from build123d import *

# Parameters (mm, degrees)
F2_W      = 200
F2_H      = 529.5
F2_H_2    = 170
F2_H_3    = 529.5044031185
F3_DEPTH  = 60
F4_R      = 260
F5_DEPTH  = 90
F6_R      = 170
F7_DEPTH  = 25
F8_R      = 280
F9_DEPTH  = 15
F10_R     = 111
F11_DEPTH = 100
F12_R     = 150
F13_DEPTH = 8
F14_R     = 5
F15_DEPTH = 25
F16_R     = 100
F17_DEPTH = 200
F18_R     = 50
F19_DEPTH = 1000
F20_R     = 112.5
F20_R_2   = 99
F21_DEPTH = 100
F22_R     = 45
F23_DEPTH = 850
F25_R     = 100
F26_DEPTH = 10
F27_R     = 64.1521691024
F27_R_2   = 45
F28_DEPTH = 15
F29_R     = 9
F30_DEPTH = 25
F31_R     = 32.5
F32_DEPTH = 850
F34_R     = 82.5
F34_R_2   = 7
F35_DEPTH = 10
F36_R     = 50
F37_DEPTH = 25


with BuildPart() as f1:
    # F0 (on Front) → F1 (revolve)
    with BuildSketch(Plane.XZ):
        Polygon((0, 1515), (0, 0), (750, 0), (768.5, 0), (768.5, 5), (750, 5), (750, 1505), (773, 1505), (773, 1515), (750, 1515), align=None)
    revolve(axis=Axis((0, 0, 757.5), (0, 0, 1)))

    # F2 (on face) → F3 (join)
    with BuildSketch(Plane.XY.offset(1515)):
        Polygon((-100, 766.5), (-140, 766.5), (-140, -766.5), (-100, -766.5), (-100, -694.5), (100, -694.5), (100, -766.4955968815), (140, -766.4955968815), (140, 766.5044031185), (100, 766.5044031185), (100, 694.5044031185), (-100, 694.5044031185), align=None)
        with Locations((0, -389.75)):
            Rectangle(F2_W, F2_H, mode=Mode.SUBTRACT)
        Rectangle(F2_W, F2_H_2, mode=Mode.SUBTRACT)
        with Locations((0, 389.7522015592)):
            Rectangle(F2_W, F2_H_3, mode=Mode.SUBTRACT)
    extrude(amount=F3_DEPTH)

    # F4 (on face) → F5 (join)
    with BuildSketch(Plane.XY.offset(1515)):
        with Locations((-445, -50)):
            Circle(F4_R)
    extrude(amount=F5_DEPTH)

    # F6 (on face) → F7 (join)
    with BuildSketch(Plane.XY.offset(1515)):
        with Locations((-350, 425)):
            Circle(F6_R)
    extrude(amount=F7_DEPTH)

    # F8 (on face) → F9 (join)
    with BuildSketch(Plane.XY.offset(1605)):
        with Locations((-445, -50)):
            Circle(F8_R)
    extrude(amount=F9_DEPTH)

    # F10 (on face) → F11 (join)
    with BuildSketch(Plane.XY.offset(1515)):
        with Locations((350, 425)):
            Circle(F10_R)
    extrude(amount=F11_DEPTH)

    # F12 (on face) → F13 (join)
    with BuildSketch(Plane.XY.offset(1615)):
        with Locations((350, 425)):
            Circle(F12_R)
    extrude(amount=F13_DEPTH)

    # F14 (on face) → F15 (cut)
    with BuildSketch(Plane.XY.offset(1623)):
        with Locations((349.8037939217, 554.9998519352)):
            Circle(F14_R)
        with Locations((220.0001480648, 424.8037939217)):
            Circle(F14_R)
        with Locations((350.1962060783, 295.0001480648)):
            Circle(F14_R)
        with Locations((479.9998519352, 425.1962060783)):
            Circle(F14_R)
    extrude(amount=-F15_DEPTH, mode=Mode.SUBTRACT)

    # F16 (on face) → F17 (cut)
    with BuildSketch(Plane.XY.offset(1623)):
        with Locations((350, 425)):
            Circle(F16_R)
    extrude(amount=-F17_DEPTH, mode=Mode.SUBTRACT)

    # F18 (on face) → F19 (cut)
    with BuildSketch(Plane.XY.offset(1515)):
        Circle(F18_R)
    extrude(amount=-F19_DEPTH, mode=Mode.SUBTRACT)

    # F20 (on face) → F21 (join)
    with BuildSketch(Plane.XY.offset(1515)):
        with Locations((-315, -451)):
            Circle(F20_R)
        with Locations((-315, -451)):
            Circle(F20_R_2, mode=Mode.SUBTRACT)
    extrude(amount=F21_DEPTH)

    # F22 (on Right) → F23 (join)
    with BuildSketch(Plane.YZ):
        with Locations((0, 133)):
            Circle(F22_R)
    extrude(amount=F23_DEPTH)

    # F25 (on offset) → F26 (join)
    with BuildSketch(Plane.YZ.offset(825)):
        with Locations((0, 133)):
            Circle(F25_R)
    extrude(amount=F26_DEPTH)

    # F27 (on face) → F28 (join)
    with BuildSketch(Plane.YZ.offset(835)):
        with Locations((0, 133)):
            Circle(F27_R)
        with Locations((0, 133)):
            Circle(F27_R_2, mode=Mode.SUBTRACT)
    extrude(amount=F28_DEPTH)

    # F29 (on face) → F30 (cut)
    with BuildSketch(Plane.YZ.offset(835)):
        with Locations((0, 217.1521691024)):
            Circle(F29_R)
        with Locations((-84.1521691024, 133)):
            Circle(F29_R)
        with Locations((0, 48.8478308976)):
            Circle(F29_R)
        with Locations((84.1521691024, 133)):
            Circle(F29_R)
    extrude(amount=-F30_DEPTH, mode=Mode.SUBTRACT)

    # F31 (on Front) → F32 (join)
    with BuildSketch(Plane.XZ):
        with Locations((0, 1400)):
            Circle(F31_R)
    extrude(amount=-F32_DEPTH)

    # F34 (on offset) → F35 (join)
    with BuildSketch(Plane(origin=(0, 825, 0), x_dir=(-1, 0, 0), z_dir=(0, 1, 0))):
        with Locations((0, 1400)):
            Circle(F34_R)
        with Locations((0, 1337.5)):
            Circle(F34_R_2, mode=Mode.SUBTRACT)
        with Locations((-62.5, 1400)):
            Circle(F34_R_2, mode=Mode.SUBTRACT)
        with Locations((62.5, 1400)):
            Circle(F34_R_2, mode=Mode.SUBTRACT)
        with Locations((0, 1462.5)):
            Circle(F34_R_2, mode=Mode.SUBTRACT)
    extrude(amount=F35_DEPTH)

    # F36 (on face) → F37 (join)
    with BuildSketch(Plane(origin=(0, 850, 0), x_dir=(-1, 0, 0), z_dir=(0, 1, 0))):
        with Locations((0, 1400)):
            Circle(F36_R)
    extrude(amount=-F37_DEPTH)


solid = f1.part
Geometry: final body of the model. Coordinates: model frame, mm. A direction names the side the tool comes from. Round coordinates to 2 decimals unless told otherwise and drop trailing zeros. Order: outer loops, then holes, each group sorted by start corner. A loop starts at its lowest first (then second) coordinate and runs counter-clockwise, first axis right, second up.
Q1. Mould query, pull axis Z, two halves, no side actions, for faces 5 (the face through (-1, 654.504, 1545)), 6 (the face through (261.914, 357.458, 1564.3)), 7 (the face through (15, 786.62, 1371.17)), 8 (the face through (-316, -450, 1515)). Classes: released by +Z, released by -Z, zero draft, split by the parting line, or undercut.
Result sheet:
face 5: zero draft
face 6: undercut
face 7: undercut
face 8: released by +Z
Q2. Section A-A, the plane y = -506.5. Output: boundary loops of the cut face in (x, z).
Result sheet:
outline: (-583.94, 1505) - (-553.13, 1505) - (-553.13, 5) - (-577.97, 5) - (-577.97, 0) - (577.97, 0) - (577.97, 5) - (553.13, 5) - (553.13, 1505) - (583.94, 1505) - (583.94, 1515) - (140, 1515) - (140, 1575) - (100, 1575) - (100, 1515) - (-100, 1515) - (-100, 1575) - (-140, 1575) - (-140, 1515) - (-217.14, 1515) - (-217.14, 1615) - (-233.02, 1615) - (-233.02, 1515) - (-396.98, 1515) - (-396.98, 1615) - (-412.86, 1615) - (-412.86, 1515) - (-583.94, 1515) - close
Q3. Access query for faces 1 (the face through (-1, 85, 1545)), 2 (the face through (786.29, -5.858, 177.617)), 3 (the face through (-1, -733, 1515)), 4 (the face through (-100, 730, 1545)). Directions: +Z, -Z, +X, -X, +Y, -Y. A direction counts if a zero-diameter tool reaches every point of the face in a straight line with its end or side. Return the directions, or none.
Result sheet:
face 1: +Z
face 2: none
face 3: +Z, -Y
face 4: +Z, +Y
Q4. Pin query (flat end, axial travel): pin 1 (2 mm diameter, centred on x = -383, y = 347, fed in from +Z); pin 2 (4 mm diameter, centred on x = 115.5, y = 214, fed in from +Z); pin 3 (12 mm diameter, centred on y = 520.5, z = 163, fed in from -X). Return the tip coordinate at first contact, or that it passes through.
Result sheet:
pin 1: stops at z = 1540
pin 2: stops at z = 1575
pin 3: stops at x = -545.7
Q5. Section C-C, the plane z = 811. Output: boundary loops of the cut face in (x, y).
Result sheet:
outline: circle Ø1500 at (0, 0); hole circle Ø100 at (0, 0)
Q6. Material intervals for probe 1 along Z at (x, y) = (0, 829); probe 2 along X at (y, z) = (-566.5, 1535); probe 3 along Z at (x, y) = (212, 430), sorted ascending.
Result sheet:
probe 1: z = 1317.5 to 1330.5, 1344.5 to 1455.5, 1469.5 to 1482.5
probe 2: x = -140 to -100, 100 to 140
probe 3: z = 0 to 1515, 1615 to 1623
Q7. Section D-D, the plane z = 304. Output: boundary loops of the cut face in (x, y), and give its area (3 significant figures).
Result sheet:
outline: circle Ø1500 at (0, 0)
area: 1,770,000 mm2
